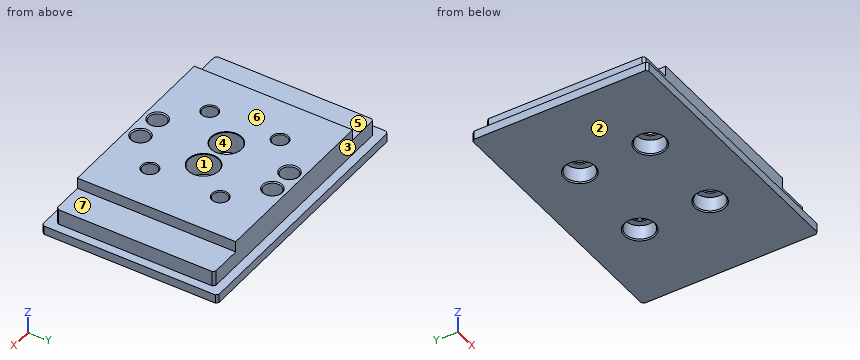
from build123d import *

# Parameters (mm, degrees)
SKETCH_1_W                        = 60
SKETCH_1_H                        = 40
EXTRUDE_1_DEPTH                   = 8
SKETCH_2_OUTSIDE_W                = 76.51
SKETCH_2_OUTSIDE_H                = 56.51
SKETCH_2_OUTSIDE_W_2              = 56
SKETCH_2_OUTSIDE_H_2              = 36
CUT_EXTRUDE_1_DEPTH               = 6
CHAMFER_1_SIZE                    = 0.5
HOLE_WIZARD_4_0_4_1_D             = 4
HOLE_WIZARD_4_0_4_1_DEPTH         = 4.5
HOLE_WIZARD_4_0_4_1_CSINK_D       = 4.5
HOLE_WIZARD_4_0_4_1_CSINK_ANGLE   = 90
HOLE_WIZARD_4_0_4_1_TIP           = 1.201721238
HOLE_WIZARD_M31_AT_2_COUNT        = 2
HOLE_WIZARD_M31_AT_2_PITCH        = 21
HOLE_WIZARD_M31_AT_3_COUNT        = 2
HOLE_WIZARD_M31_AT_3_PITCH        = 26.400757565
HOLE_WIZARD_M31_AT_4_COUNT        = 2
HOLE_WIZARD_M31_AT_4_PITCH        = 16
SKETCH_7_W                        = 7.5
SKETCH_7_H                        = 2.5
CUT_EXTRUDE_2_DEPTH               = 21
CUT_EXTRUDE_2_DEPTH_BACK          = 21
HOLE_WIZARD_6_8_6_8_1_D           = 6.8
HOLE_WIZARD_6_8_6_8_1_DEPTH       = 5
HOLE_WIZARD_6_8_6_8_1_CSINK_D     = 7
HOLE_WIZARD_6_8_6_8_1_CSINK_ANGLE = 90
HOLE_WIZARD_6_8_6_8_1_TIP         = 2.042926105


with BuildPart() as part:
    # Эскиз1 → Бобышка-Вытянуть1 (new body)
    with BuildSketch(Plane.XY):
        Rectangle(SKETCH_1_W, SKETCH_1_H)
    extrude(amount=EXTRUDE_1_DEPTH)

    # Эскиз2 outside → Вырез-Вытянуть1 (cut)
    with BuildSketch(Plane.XY.offset(8)):
        Rectangle(SKETCH_2_OUTSIDE_W, SKETCH_2_OUTSIDE_H)
        Rectangle(SKETCH_2_OUTSIDE_W_2, SKETCH_2_OUTSIDE_H_2, mode=Mode.SUBTRACT)
    extrude(amount=-CUT_EXTRUDE_1_DEPTH, mode=Mode.SUBTRACT)

    # Фаска1
    chamfer_1_edges = [part.edges().sort_by_distance(p)[0] for p in [
        (30, -20, 1),
        (-30, -20, 1),
        (-30, 20, 1),
        (30, 20, 1),
        (28, -18, 5),
        (-28, -18, 5),
        (-28, 18, 5),
        (28, 18, 5),
    ]]
    chamfer(chamfer_1_edges, length=CHAMFER_1_SIZE)

    # Диаметр отверстия Ø4.0 (4)1
    with Locations(Plane.XY.offset(8)):
        with Locations((-3, -15), (3, -15), (3, 15), (-3, 15)):
            CounterSinkHole(HOLE_WIZARD_4_0_4_1_D / 2, HOLE_WIZARD_4_0_4_1_CSINK_D / 2, depth=HOLE_WIZARD_4_0_4_1_DEPTH, counter_sink_angle=HOLE_WIZARD_4_0_4_1_CSINK_ANGLE)
            with Locations((0, 0, -(HOLE_WIZARD_4_0_4_1_DEPTH + HOLE_WIZARD_4_0_4_1_TIP / 2))):  # 118° drill point
                Cone(0, HOLE_WIZARD_4_0_4_1_D / 2, HOLE_WIZARD_4_0_4_1_TIP, mode=Mode.SUBTRACT)

    # Эскиз5 → Цековка для винта с внутренним шестигранником M31 (revolve, cut)
    with BuildSketch(Plane(origin=(10.5, 8, 0), x_dir=(0, 1, 0), z_dir=(1, 0, 0))):
        Polygon((0, 0), (0, 8), (1.9, 8), (1.7, 7.8), (1.7, 3.7), (1.9, 3.5), (3.25, 3.5), (3.25, 0.25), (3.5, 0), align=None)
    hole_wizard_m31 = revolve(axis=Axis((10.5, 8, -6.35), (0, 0, 1)), mode=Mode.SUBTRACT)

    # Цековка для винта с внутренним шестигранником M31 at 2: Цековка для винта с внутренним шестигранником M31 ×2
    with Locations(*[(-i * HOLE_WIZARD_M31_AT_2_PITCH, 0, 0) for i in range(1, HOLE_WIZARD_M31_AT_2_COUNT)]):
        add(hole_wizard_m31, mode=Mode.SUBTRACT)

    # Цековка для винта с внутренним шестигранником M31 at 3: Цековка для винта с внутренним шестигранником M31 ×2
    with Locations(*[Vector(-0.79543172, -0.606043215, 0) * (i * HOLE_WIZARD_M31_AT_3_PITCH) for i in range(1, HOLE_WIZARD_M31_AT_3_COUNT)]):
        add(hole_wizard_m31, mode=Mode.SUBTRACT)

    # Цековка для винта с внутренним шестигранником M31 at 4: Цековка для винта с внутренним шестигранником M31 ×2
    with Locations(*[(0, -i * HOLE_WIZARD_M31_AT_4_PITCH, 0) for i in range(1, HOLE_WIZARD_M31_AT_4_COUNT)]):
        add(hole_wizard_m31, mode=Mode.SUBTRACT)

    # Эскиз7 → Вырез-Вытянуть2 (cut, two sides)
    with BuildSketch(Plane(origin=(0, 0, 0), x_dir=(1, 0, 0), z_dir=(0, 1, 0))) as cut_extrude_2_sk:
        with Locations((24.25, -6.75)):
            Rectangle(SKETCH_7_W, SKETCH_7_H)
        with Locations((-24.25, -6.75)):
            Rectangle(SKETCH_7_W, SKETCH_7_H)
    extrude(amount=CUT_EXTRUDE_2_DEPTH, mode=Mode.SUBTRACT)
    extrude(cut_extrude_2_sk.sketch, amount=-CUT_EXTRUDE_2_DEPTH_BACK, mode=Mode.SUBTRACT)

    # Диаметр отверстия Ø6.8 (6.8)1
    with Locations(Plane.XY.offset(8)):
        with Locations((4, 0), (-4, 0)):
            CounterSinkHole(HOLE_WIZARD_6_8_6_8_1_D / 2, HOLE_WIZARD_6_8_6_8_1_CSINK_D / 2, depth=HOLE_WIZARD_6_8_6_8_1_DEPTH, counter_sink_angle=HOLE_WIZARD_6_8_6_8_1_CSINK_ANGLE)
            with Locations((0, 0, -(HOLE_WIZARD_6_8_6_8_1_DEPTH + HOLE_WIZARD_6_8_6_8_1_TIP / 2))):  # 118° drill point
                Cone(0, HOLE_WIZARD_6_8_6_8_1_D / 2, HOLE_WIZARD_6_8_6_8_1_TIP, mode=Mode.SUBTRACT)


solid = part.part
Can you work these out from the model? Positions are in its coordinate system, mm. Face numbers are marked on the shaded views. A direction names the side the tool comes from. Round coordinates to 2 decimals unless told otherwise and drop trailing zeros. Write each loop counter-clockwise with the first axis right and the second up, starting at its lowest first coordinate (ties: lowest second). Pieces come first, ordered by that corner, then holes. Notation, with made-up numbers: (-36, -4.75) - (18, -4.75) arc R28 cw to (18, 23.25) - close; hole circle Ø10 at (-13.5, 58). An arc over 180 degrees is marked (long way). Write each question's results on one line, items separated by ' | '. Start each with the question number.
1) Which directions (+Z, -Z, +X, -X, +Y, -Y) give clear straight access to the entire face, cutting with the end or side of a thin tool? Please do the marked faces 4, 5, 6 and 7.
2) Suppose I cut it at A-A (z = 7). Give the number of separate pieces and of enclosed holes in the cut face, and give its area (3 significant figures).
3) Please list where these lines run through material, in increasing order: line 1 (X direction, y = -8, z = 4.65); line 2 (X direction, y = 8, z = 1.2); line 3 (Y direction, x = -3, z = 4.75).
4) For pin 1 Ø6 at (x, y) = (-10.5, 8) entering from -Z; pin 2 Ø7 at (x, y) = (11.5, 9) entering from -Z; pin 3 Ø4 at (x, z) = (-6, 6) entering from +Y; pin 4 Ø3 at (x, y) = (-10.5, 8) entering from +Z, each with a flat end and sliding along its axis, tell me the tip position at first contact or that it passes through.
5) We'd pull the mould along Y, two halves only. Please class the marked faces 1, 2 and 3: released by +Y, released by -Y, zero draft, split by the parting line, or undercut.
6) Suppose I cut it at B-B (x = 17.5). List the corners of the cut face in (y, z) for me.
Here are the results:
1) face 4: +Z | face 5: +Z, -X, +Y, -Y | face 6: +Z, +X, -X, +Y, -Y | face 7: +Z, +X, +Y, -Y
2) separate pieces: 1 | enclosed holes: 10 | area: 1,320 mm2
3) line 1: x = -28 to -12.2, -8.8 to 8.8, 12.2 to 28 | line 2: x = -30 to -13.75, -7.25 to 7.25, 13.75 to 30 | line 3: y = -18 to -17, -13 to -3.25, 3.25 to 13, 17 to 18
4) pin 1: stops at z = 3.5 | pin 2: stops at z = 0 | pin 3: stops at y = 18 | pin 4: passes through
5) face 1: undercut | face 2: zero draft | face 3: released by +Y
6) outline: (-20, 0) - (20, 0) - (20, 2) - (18, 2) - (18, 8) - (-18, 8) - (-18, 2) - (-20, 2) - close
